Verification items for the finished model (mm, model axes). A direction names the side the tool comes from. Coordinates: 2 decimals unless noted, no trailing zeros. Write each loop counter-clockwise with the first axis right and the second up, starting at its lowest first coordinate (ties: lowest second). Pieces come first, ordered by that corner, then holes. Notation, with made-up numbers: (12, 34.25) -> (41, 34.25) arc R12 ccw to (41, 54.25) -> close; hole circle Ø8 at (23, 83). An arc over 180 degrees is marked (long way). Answer in a Markdown table with one row per item.
Autodesk Inventor part; units mm, degrees
ref_plane "YZ Plane" through (0, 0, 0) normal (1, 0, 0) x (0, 1, 0)
ref_plane "XZ Plane" through (0, 0, 0) normal (0, 1, 0) x (-1, 0, 0)
ref_plane "XY Plane" through (0, 0, 0) normal (0, 0, 1) x (1, 0, 0)
sketch "Sketch1" plane through (0, 0, 0) normal (1, 0, 0) x (0, 1, 0)
  line L0 (0, 0) -> (69.85, 0)
  line L1 (69.85, 0) -> (69.85, -150.4)
  line L2 (69.85, -150.4) -> (0, -150.4)
  line L3 (0, -150.4) -> (0, 0)
  dimension "d0" = 69.85
  dimension "d1" = 150.4
extrude "Extrusion1" add sketch "Sketch1" along normal blind 2
sketch "Sketch2" plane through (2, 0, 0) normal (1, 0, 0) x (0, 0, -1)
  line L0 (150.4, 0) -> (150.4, 69.85)
  line L1 (150.4, 69.85) -> (0, 69.85)
  line L2 (0, 69.85) -> (0, 0)
  line L3 (0, 0) -> (150.4, 0)
  line L4 (150.4, 69.85) -> (148.4, 69.85)
  line L5 (148.4, 69.85) -> (148.4, 0)
  line L6 (148.4, 0) -> (150.4, 0)
  line L7 (150.4, 0) -> (150.4, 69.85)
  line L8 (0, 69.85) -> (2, 69.85)
  line L9 (2, 69.85) -> (2, 0)
  line L10 (2, 0) -> (0, 0)
  line L11 (0, 0) -> (0, 69.85)
  line L12 (0, 0) -> (150.4, 0)
  line L13 (150.4, 0) -> (150.4, 2)
  line L14 (150.4, 2) -> (0, 2)
  line L15 (0, 2) -> (0, 0)
  point P0 (2, 2)
  point P1 (148.4, 2)
  dimension "d4" = 2
  dimension "d5" = 2
  dimension "d6" = 2
extrude "Extrusion2" add sketch "Sketch2" along normal blind 2 contours L14 L9 L1 L5
sketch "Sketch3" plane through (4, 0, 0) normal (1, 0, 0) x (0, 0, -1)
  line L0 (150.4, 0) -> (150.4, 69.85)
  line L1 (0, 0) -> (150.4, 0)
  line L2 (0, 69.85) -> (0, 0)
  line L3 (150.4, 69.85) -> (0, 69.85)
  line L4 (0, 69.85) -> (75.2, 69.85) construction
  line L5 (75.2, 69.85) -> (75.2, 0) construction
  line L6 (75.2, 0) -> (0, 0) construction
  line L7 (0, 0) -> (0, 69.85) construction
  line L8 (0, 0) -> (150.4, 0) construction
  line L9 (0, 0) -> (37.6, 0) construction
  line L10 (37.6, 0) -> (37.6, 69.85) construction
  line L11 (37.6, 69.85) -> (0, 69.85) construction
  line L12 (0, 69.85) -> (0, 0) construction
  line L13 (150.4, 0) -> (150.4, 69.85) construction
  line L14 (75.2, 69.85) -> (150.4, 69.85) construction
  line L15 (150.4, 69.85) -> (150.4, 0) construction
  line L16 (150.4, 0) -> (75.2, 0) construction
  line L17 (75.2, 0) -> (75.2, 69.85) construction
  line L18 (75.2, 0) -> (112.8, 0) construction
  line L19 (112.8, 0) -> (112.8, 69.85) construction
  line L20 (112.8, 69.85) -> (75.2, 69.85) construction
  line L21 (75.2, 69.85) -> (75.2, 0) construction
  line L22 (34.425, 0) -> (34.425, 69.85) construction
  line L23 (34.425, 69.85) -> (40.775, 69.85) construction
  line L24 (40.775, 69.85) -> (40.775, 0) construction
  line L25 (40.775, 0) -> (34.425, 0) construction
  line L26 (34.425, 0) -> (40.775, 69.85) construction
  line L27 (34.425, 69.85) -> (40.775, 0) construction
  line L28 (72.025, 0) -> (72.025, 69.85) construction
  line L29 (72.025, 69.85) -> (78.375, 69.85) construction
  line L30 (78.375, 69.85) -> (78.375, 0) construction
  line L31 (78.375, 0) -> (72.025, 0) construction
  line L32 (72.025, 0) -> (78.375, 69.85) construction
  line L33 (72.025, 69.85) -> (78.375, 0) construction
  line L34 (109.625, 0) -> (109.625, 69.85) construction
  line L35 (109.625, 69.85) -> (115.975, 69.85) construction
  line L36 (115.975, 69.85) -> (115.975, 0) construction
  line L37 (115.975, 0) -> (109.625, 0) construction
  line L38 (109.625, 0) -> (115.975, 69.85) construction
  line L39 (109.625, 69.85) -> (115.975, 0) construction
  line L40 (34.425, 69.85) -> (40.775, 69.85)
  line L41 (40.775, 69.85) -> (40.775, 0)
  line L42 (40.775, 0) -> (34.425, 0)
  line L43 (34.425, 0) -> (34.425, 69.85)
  line L44 (72.025, 0) -> (78.375, 0)
  line L45 (78.375, 0) -> (78.375, 69.85)
  line L46 (78.375, 69.85) -> (72.025, 69.85)
  line L47 (72.025, 69.85) -> (72.025, 0)
  line L48 (109.625, 69.85) -> (115.975, 69.85)
  line L49 (115.975, 69.85) -> (115.975, 0)
  line L50 (115.975, 0) -> (109.625, 0)
  line L51 (109.625, 0) -> (109.625, 69.85)
  point P0 (37.6, 34.925)
  point P1 (75.2, 34.925)
  point P2 (112.8, 34.925)
  dimension "d9" = 6.35
  dimension "d10" = 6.35
  dimension "d11" = 6.35
extrude "Extrusion3" add sketch "Sketch3" along normal blind 4 contours L1 L51 L3 L49 | L1 L47 L3 L45 | L1 L43 L3 L41
sketch "Sketch4" plane through (0, 69.85, 0) normal (0, 1, 0) x (1, 0, 0)
  line L0 (0, 150.4) -> (0, 0)
  line L1 (0, 150.4) -> (0, 0) construction
  line L2 (0, 0) -> (2, 0) construction
  line L3 (2, 2) -> (2, 0) construction
  line L4 (2, 2) -> (4, 2) construction
  line L5 (4, 34.425) -> (4, 2) construction
  line L6 (4, 34.425) -> (8, 34.425) construction
  line L7 (8, 40.775) -> (8, 34.425) construction
  line L8 (4, 40.775) -> (8, 40.775) construction
  line L9 (4, 72.025) -> (4, 40.775) construction
  line L10 (4, 72.025) -> (8, 72.025) construction
  line L11 (8, 78.375) -> (8, 72.025) construction
  line L12 (4, 78.375) -> (8, 78.375) construction
  line L13 (4, 109.625) -> (4, 78.375) construction
  line L14 (4, 109.625) -> (8, 109.625) construction
  line L15 (8, 115.975) -> (8, 109.625) construction
  line L16 (4, 115.975) -> (8, 115.975) construction
  line L17 (4, 148.4) -> (4, 115.975) construction
  line L18 (2, 148.4) -> (4, 148.4) construction
  line L19 (2, 150.4) -> (2, 148.4) construction
  line L20 (0, 150.4) -> (2, 150.4) construction
  line L21 (2, 0) -> (0, 0)
  line L22 (0, 0) -> (0, 150.4)
  line L23 (0, 150.4) -> (2, 150.4)
  line L24 (2, 150.4) -> (2, 0)
  line L25 (2, 0) -> (8, 0)
  line L26 (8, 0) -> (8, 150.4)
  line L27 (8, 150.4) -> (2, 150.4)
  line L28 (2, 150.4) -> (2, 0)
extrude "Extrusion4" cut sketch "Sketch4" against normal blind 2 contours L27 L26 L25 L24
sketch "Sketch5" plane through (0, 67.85, 0) normal (0, 1, 0) x (1, 0, 0)
  line L0 (4, 115.975) -> (8, 115.975)
  line L1 (4, 148.4) -> (4, 115.975)
  line L2 (2, 148.4) -> (4, 148.4)
  line L3 (2, 2) -> (2, 148.4)
  line L4 (4, 2) -> (2, 2)
  line L5 (4, 34.425) -> (4, 2)
  line L6 (8, 34.425) -> (4, 34.425)
  line L7 (8, 40.775) -> (8, 34.425)
  line L8 (4, 40.775) -> (8, 40.775)
  line L9 (4, 72.025) -> (4, 40.775)
  line L10 (8, 72.025) -> (4, 72.025)
  line L11 (8, 78.375) -> (8, 72.025)
  line L12 (4, 78.375) -> (8, 78.375)
  line L13 (4, 109.625) -> (4, 78.375)
  line L14 (8, 109.625) -> (4, 109.625)
  line L15 (8, 115.975) -> (8, 109.625)
  line L16 (2, 2) -> (4, 2)
  line L17 (2, 2) -> (8, 2)
  line L18 (8, 2) -> (8, 148.4)
  line L19 (8, 148.4) -> (2, 148.4)
  line L20 (2, 148.4) -> (2, 2)
  point P0 (0, 0)
  point P1 (4, 2)
extrude "Extrusion5" add sketch "Sketch5" against normal blind 2 contours L1 L19 L18 L0 | L18 L12 L13 L14 | L18 L8 L9 L10 | L5 L6 L18 L17
sketch "Sketch6" plane through (4, 0, 0) normal (1, 0, 0) x (0, 0, -1)
  line L0 (2, 67.85) -> (148.4, 67.85) construction
  line L1 (2, 67.85) -> (2, 65.85) construction
  line L2 (34.425, 65.85) -> (2, 65.85) construction
  line L3 (34.425, 65.85) -> (34.425, 0) construction
  line L4 (34.425, 0) -> (40.775, 0) construction
  line L5 (40.775, 0) -> (40.775, 65.85) construction
  line L6 (72.025, 65.85) -> (40.775, 65.85) construction
  line L7 (72.025, 65.85) -> (72.025, 0) construction
  line L8 (72.025, 0) -> (78.375, 0) construction
  line L9 (78.375, 0) -> (78.375, 65.85) construction
  line L10 (109.625, 65.85) -> (78.375, 65.85) construction
  line L11 (109.625, 65.85) -> (109.625, 0) construction
  line L12 (109.625, 0) -> (115.975, 0) construction
  line L13 (115.975, 0) -> (115.975, 65.85) construction
  line L14 (148.4, 65.85) -> (115.975, 65.85) construction
  line L15 (148.4, 67.85) -> (148.4, 65.85) construction
  line L16 (109.625, 65.85) -> (78.375, 65.85) construction
  line L17 (78.375, 65.85) -> (78.375, 2) construction
  line L18 (78.375, 2) -> (109.625, 2) construction
  line L19 (109.625, 2) -> (109.625, 65.85) construction
  line L20 (148.4, 65.85) -> (115.975, 65.85) construction
  line L21 (115.975, 65.85) -> (115.975, 2) construction
  line L22 (115.975, 2) -> (148.4, 2) construction
  line L23 (148.4, 2) -> (148.4, 65.85) construction
  line L24 (72.025, 65.85) -> (40.775, 65.85) construction
  line L25 (40.775, 65.85) -> (40.775, 2) construction
  line L26 (40.775, 2) -> (72.025, 2) construction
  line L27 (72.025, 2) -> (72.025, 65.85) construction
  line L28 (78.375, 2) -> (78.375, 28.67) construction
  line L29 (94, 28.67) -> (114.32, 28.67)
  line L30 (114.32, 28.67) -> (73.68, 28.67)
  line L31 (73.68, 28.67) -> (67.33, 28.67)
  line L32 (67.33, 28.67) -> (80.03, 28.67)
  line L33 (80.03, 28.67) -> (80.03, 34.67)
  line L34 (80.03, 34.67) -> (67.33, 34.67)
  line L35 (67.33, 34.67) -> (67.33, 28.67)
  line L36 (114.32, 28.67) -> (120.67, 28.67)
  line L37 (120.67, 28.67) -> (107.97, 28.67)
  line L38 (107.97, 28.67) -> (107.97, 34.67)
  line L39 (107.97, 34.67) -> (120.67, 34.67)
  line L40 (120.67, 34.67) -> (120.67, 28.67)
  point P0 (0, 0)
  dimension "d18" = 26.67
  dimension "d31" = 20.32
  dimension "d32" = 40.64
  dimension "d33" = 6.35
  dimension "d34" = 12.7
  dimension "d35" = 6
  dimension "d36" = 6.35
  dimension "d37" = 12.7
  dimension "d38" = 6
extrude "Extrusion6" add sketch "Sketch6" along normal blind 33.02
sketch "Sketch12" plane through (4, 34.67, -67.33) normal (0, 1, 0) x (1, 0, 0)
  line L0 (4, 11.045) -> (0, 11.045) construction
  line L1 (4, 4.695) -> (4, 11.045) construction
  line L2 (0, 4.695) -> (4, 4.695) construction
  line L3 (0, 0) -> (0, 4.695) construction
  line L4 (0, 0) -> (33.02, 0) construction
  line L5 (33.02, 12.7) -> (33.02, 0) construction
  line L6 (0, 12.7) -> (33.02, 12.7) construction
  line L7 (0, 11.045) -> (0, 12.7) construction
  line L8 (4, 48.645) -> (0, 48.645) construction
  line L9 (4, 42.295) -> (4, 48.645) construction
  line L10 (0, 42.295) -> (4, 42.295) construction
  line L11 (0, 40.64) -> (0, 42.295) construction
  line L12 (0, 40.64) -> (33.02, 40.64) construction
  line L13 (33.02, 53.34) -> (33.02, 40.64) construction
  line L14 (0, 53.34) -> (33.02, 53.34) construction
  line L15 (0, 48.645) -> (0, 53.34) construction
  line L16 (4, 4.695) -> (4, -26.555) construction
  line L17 (4, 4.695) -> (33.02, 4.695) construction
  line L18 (33.02, 4.695) -> (33.02, 0) construction
  line L19 (33.02, 0) -> (4, 0) construction
  line L20 (4, 0) -> (4, 4.695) construction
  circle A0 centre (18.51, 6.35) radius 2.25 construction
  line L21 (4, 48.645) -> (33.02, 48.645) construction
  circle A1 centre (18.51, 46.99) radius 2.25 construction
  circle A2 centre (18.51, 6.35) radius 2.25
  circle A3 centre (18.51, 46.99) radius 2.25
  point P0 (-4, -67.33)
  dimension "d39" = 4.5
  dimension "d40" = 4.5
extrude "Extrusion10" cut sketch "Sketch12" against normal blind 5
properties part number "leftwall"
1. Section check A-A, the plane x = 22.51. Record the boundary of the cut face in (y, z), plus the area to 3 significant figures.
Geometry says:
| item | result |
|---|---|
| outline | (28.67, -120.67) -> (34.67, -120.67) -> (34.67, -116.57) -> (29.67, -116.57) -> (29.67, -112.07) -> (34.67, -112.07) -> (34.67, -107.97) -> (28.67, -107.97) -> close; (28.67, -80.03) -> (34.67, -80.03) -> (34.67, -75.93) -> (29.67, -75.93) -> (29.67, -71.43) -> (34.67, -71.43) -> (34.67, -67.33) -> (28.67, -67.33) -> close |
| area | 107 mm^2 |
2. Mould release check, pull along Y, two halves, no side actions. Record for faces 1 (the flat face through (5, 67.85, -76)), 2 (the flat face through (6, 50, -115.975)), 3 (the flat face through (20, 32, -120.67)): released by +Y, released by -Y, zero draft, split by the parting line, or undercut.
Geometry says:
| item | result |
|---|---|
| face 1 | released by +Y |
| face 2 | undercut |
| face 3 | zero draft |
3. Thickness scan on line 1 (Z direction, x = 22.51, y = 31.3); line 2 (X direction, y = 31, z = -114); line 3 (Z direction, x = 22, y = 31). Record the ranges inside material, lowest first. Write a range as from..to.
Geometry says:
| item | result |
|---|---|
| line 1 | -120.67..-116.57, -112.07..-107.97, -80.03..-75.93, -71.43..-67.33 |
| line 2 | 0..20.28, 24.74..37.02 |
| line 3 | -120.67..-116.51, -112.13..-107.97, -80.03..-75.87, -71.49..-67.33 |
4. Tool access check on faces 4 (the flat face through (6, 14, -109.625)), 5 (the flat face through (6, 50, -78.375)), 6 (the flat face through (8, 15, -113)), 7 (the cylindrical face through (22.22, 32.2, -116.55)). Record the directions out of +Z, -Z, +X, -X, +Y, -Y that give a thin tool (end or side, any length) a straight path to the whole face; none if there is none.
Geometry says:
| item | result |
|---|---|
| face 4 | +X, -Y |
| face 5 | +X |
| face 6 | +Z, -Z, +X, -Y |
| face 7 | +Y |
5. Section check B-B, the plane y = 15.5. Record the boundary of the cut face in (x, z) (3 decimals).
Geometry says:
| item | result |
|---|---|
| outline | (0, -150.4) -> (2, -150.4) -> (2, -148.4) -> (4, -148.4) -> (4, -115.975) -> (8, -115.975) -> (8, -109.625) -> (4, -109.625) -> (4, -78.375) -> (8, -78.375) -> (8, -72.025) -> (4, -72.025) -> (4, -40.775) -> (8, -40.775) -> (8, -34.425) -> (4, -34.425) -> (4, -2) -> (2, -2) -> (2, 0) -> (0, 0) -> close |
6. Section check C-C, the plane z = -114.32. Record the boundary of the cut face in (x, y), plus the area to 3 significant figures.
Geometry says:
| item | result |
|---|---|
| outline | (0, 0) -> (2, 0) -> (2, 2) -> (4, 2) -> (4, 0) -> (8, 0) -> (8, 28.67) -> (37.02, 28.67) -> (37.02, 34.67) -> (24.76, 34.67) -> (24.76, 29.67) -> (20.26, 29.67) -> (20.26, 34.67) -> (8, 34.67) -> (8, 67.85) -> (2, 67.85) -> (2, 69.85) -> (0, 69.85) -> close |
| area | 694 mm^2 |
7. Depth check by flat-ended pin: P1, Ø1.6, axis at x = 3.5, z = -85, coming from the -Y side; P2, Ø6.5, axis at x = 5.5, y = 26, coming from the +Z side; P3, Ø6.5, axis at x = 14, z = -74, coming from the +Y side. Enter the tip coordinate at first touch or a pass-through.
Geometry says:
| item | result |
|---|---|
| P1 | y = 2 |
| P2 | z = -2 |
| P3 | y = 34.67 |
